from build123d import *

# Parameters (mm, degrees)
SKETCH1_W           = 50.8
SKETCH1_H           = 15.24
BOSS_EXTRUDE2_DEPTH = 30.48
SKETCH2_W           = 76.2
SKETCH2_H           = 15.24
BOSS_EXTRUDE3_DEPTH = 38.1
SKETCH3_W           = 50.8
SKETCH3_H           = 20.32
CUT_EXTRUDE1_DEPTH  = 80.919234231
FILLET1_R           = 5.08
FILLET4_R           = 12.7


with BuildPart() as part:
    # Sketch1 → Boss-Extrude2 (new body)
    with BuildSketch(Plane.XY):
        Rectangle(SKETCH1_W, SKETCH1_H)
    extrude(amount=BOSS_EXTRUDE2_DEPTH)

    # Sketch2 → Boss-Extrude3 (add)
    with BuildSketch(Plane.XY.offset(30.48)):
        Rectangle(SKETCH2_W, SKETCH2_H)
    extrude(amount=BOSS_EXTRUDE3_DEPTH)

    # Sketch3 → Cut-Extrude1 (cut, through all)
    with BuildSketch(Plane.XZ.offset(7.62)):
        with Locations((0, 49.167262881)):
            Rectangle(SKETCH3_W, SKETCH3_H)
    extrude(amount=-CUT_EXTRUDE1_DEPTH, mode=Mode.SUBTRACT)

    # Fillet1
    fillet1_edges = [part.edges().sort_by_distance(p)[0] for p in [
        (-25.4, 0, 39.007262881),
        (-25.4, 0, 59.327262881),
        (25.4, 0, 59.327262881),
        (25.4, 0, 39.007262881),
    ]]
    fillet(fillet1_edges, radius=FILLET1_R)

    # Fillet4
    fillet4_edges = [part.edges().sort_by_distance(p)[0] for p in [
        (38.1, 0, 30.48),
        (38.1, 0, 68.58),
        (-38.1, 0, 30.48),
        (-38.1, 0, 68.58),
    ]]
    fillet(fillet4_edges, radius=FILLET4_R - 0.0001)  # a hair under: the kernel refuses the full size


solid = part.part
Part model, mm, in its own coordinate system. A direction names the side the tool comes from. Give positions to 0.01 mm unless a question says otherwise; leave off trailing zeros. Loops run counter-clockwise (first coordinate to the right, second up) from the corner with the lowest first, then second, coordinate; pieces in that order, holes last.
(1) Pin check, flat tips, straight feed: pin 1 (1.5 mm diameter, centred on x = 26.5, y = 0.5, fed in from +Z); pin 2 (8 mm diameter, centred on y = -4, z = 8, fed in from -X). Stop position of each tip, or through.
Return value:
pin 1: stops at z = 68.58
pin 2: stops at x = -25.4
(2) Band-saw the part on D-D (z = 23). Write the cut outline in (x, y).
Return value:
outline: (-25.4, -7.62) - (25.4, -7.62) - (25.4, 7.62) - (-25.4, 7.62) - close
(3) 3-axis set-ups, long thin cutter, end or side, ignore diameter. For faces 1 (the flat face through (25.4, 0, 49)), 2 (the flat face through (-1, 7.62, 34)), 3 (the flat face through (25.4, 0, 15)): which of +Z, -Z, +X, -X, +Y, -Y reach the whole face in a straight line?
Return value:
face 1: +Y, -Y
face 2: +Z, -Z, +X, -X, +Y
face 3: -Z, +X, +Y, -Y
(4) Band-saw the part on C-C (z = 49). Write the cut outline in (x, y), and give its area (3 significant figures).
Return value:
outline: (-38.1, -7.62) - (-25.4, -7.62) - (-25.4, 7.62) - (-38.1, 7.62) - close; (25.4, -7.62) - (38.1, -7.62) - (38.1, 7.62) - (25.4, 7.62) - close
area: 387 mm2
(5) Drill centre lines: line 1 along X through (y, z) = (-6.25, 50); line 2 along Z through (x, y) = (14, -6.5); line 3 along X through (y, z) = (2, 27.5). Where is each one in solid material? Low to high.
Return value:
line 1: x = -38.1 to -25.4, 25.4 to 38.1
line 2: z = 0 to 39.01, 59.33 to 68.58
line 3: x = -25.4 to 25.4
(6) Pull direction X, two halves, no side cores. Call faces 4 (the cylindrical face through (34.48, 0.11, 34.3)), 5 (the flat face through (0, 0, 68.58)), 6 (the cylindrical face through (-23.95, 0.11, 57.8)): pulls with the +X half, pulls with the -X half, needs draft (parallel to the pull), parting line crosses it, or undercut.
Return value:
face 4: pulls with the +X half
face 5: needs draft
face 6: undercut
(7) Band-saw the part on B-B (x = 16.5). Write the cut outline in (y, z), and give its area (3 significant figures).
Return value:
outline: (-7.62, 0) - (7.62, 0) - (7.62, 39.01) - (-7.62, 39.01) - close; (-7.62, 59.33) - (7.62, 59.33) - (7.62, 68.58) - (-7.62, 68.58) - close
area: 735 mm2
